The model under review builds one solid part; all positions refer to its coordinate system, in mm. Coordinates: 2 decimals unless noted, no trailing zeros. Loops run counter-clockwise (first coordinate to the right, second up) from the corner with the lowest first, then second, coordinate; pieces in that order, holes last. Notation, with made-up numbers: M -30.75,43.5 L -6.75,43.5 A21 ccw -6.75,58.5 Z; hole C 73.25,63.25 d1. An arc over 180 degrees is marked long. Use one line per item in the form item = value.
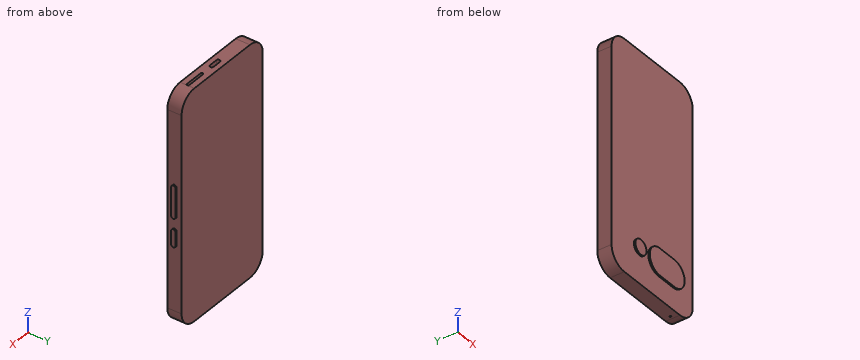
Autodesk Inventor part; units mm, degrees
ref_plane "YZ Plane" through (0, 0, 0) normal (1, 0, 0) x (0, 1, 0)
ref_plane "XZ Plane" through (0, 0, 0) normal (0, 1, 0) x (-1, 0, 0)
ref_plane "XY Plane" through (0, 0, 0) normal (0, 0, 1) x (1, 0, 0)
sketch "スケッチ1" plane through (0, 0, 0) normal (0, 1, 0) x (-1, 0, 0)
  line L0 (11.5, 0) -> (61.8, 0)
  line L1 (73.3, -11.5) -> (73.3, -143.2)
  line L2 (61.8, -154.7) -> (11.5, -154.7)
  line L3 (0, -143.2) -> (0, -11.5)
  arc A0 (73.3, -11.5) -> (61.8, 0) centre (61.8, -11.5) ccw
  arc A1 (11.5, 0) -> (0, -11.5) centre (11.5, -11.5) ccw
  arc A2 (0, -143.2) -> (11.5, -154.7) centre (11.5, -143.2) ccw
  arc A3 (61.8, -154.7) -> (73.3, -143.2) centre (61.8, -143.2) ccw
  point P0 (0, 0)
  point P1 (73.3, -154.7)
  point P2 (73.3, 0)
  point P3 (0, -154.7)
  dimension "d0" = 73.3
  dimension "d1" = 154.7
  dimension "d2" = 171.187
  dimension "d3" = 11.5
extrude "押し出し1" add sketch "スケッチ1" along normal blind 9.6
sketch "スケッチ2" plane through (-61.8, 0, 0) normal (0, 0, 1) x (1, 0, 0)
  line L0 (28.075, 6.05) -> (22.225, 6.05)
  line L1 (20.975, 4.8) -> (20.975, 4.8)
  line L2 (22.225, 3.55) -> (28.075, 3.55)
  line L3 (29.325, 4.8) -> (29.325, 4.8)
  line L4 (0, 9.6) -> (50.3, 9.6)
  line L5 (50.3, 0) -> (50.3, 9.6)
  arc A0 (22.225, 6.05) -> (20.975, 4.8) centre (22.225, 4.8) ccw
  arc A1 (20.975, 4.8) -> (22.225, 3.55) centre (22.225, 4.8) ccw
  arc A2 (28.075, 3.55) -> (29.325, 4.8) centre (28.075, 4.8) ccw
  arc A3 (29.325, 4.8) -> (28.075, 6.05) centre (28.075, 4.8) ccw
  line L6 (37.15, 5.625) -> (49.4, 5.625)
  line L7 (50.225, 4.8) -> (50.225, 4.8)
  line L8 (49.4, 3.975) -> (37.15, 3.975)
  line L9 (36.325, 4.8) -> (36.325, 4.8)
  arc A4 (50.225, 4.8) -> (49.4, 5.625) centre (49.4, 4.8) ccw
  arc A5 (49.4, 3.975) -> (50.225, 4.8) centre (49.4, 4.8) ccw
  arc A6 (37.15, 5.625) -> (36.325, 4.8) centre (37.15, 4.8) ccw
  arc A7 (36.325, 4.8) -> (37.15, 3.975) centre (37.15, 4.8) ccw
  point P0 (61.8, 0)
  point P1 (29.325, 6.05)
  point P2 (20.975, 3.55)
  point P3 (29.325, 3.55)
  point P4 (25.15, 6.05)
  point P5 (25.15, 9.6)
  point P6 (50.3, 4.8)
  point P7 (50.3, 4.8)
  point P8 (20.975, 4.8)
  point P9 (29.325, 4.8)
  point P10 (50.225, 3.975)
  point P11 (50.225, 5.625)
  point P12 (36.325, 3.975)
  point P13 (50.3, 4.8)
  point P14 (36.325, 4.8)
  point P15 (50.225, 4.8)
  dimension "d6" = 8.35
  dimension "d7" = 2.5
  dimension "d8" = 1.25
  dimension "d16" = 13.9
  dimension "d17" = 1.65
  dimension "d18" = 0.825
  dimension "d19" = 7
extrude "押し出し2" cut sketch "スケッチ2" against normal blind 5
sketch "スケッチ4" plane through (0, 0, -11.5) normal (1, 0, 0) x (0, 0, -1)
  line L0 (78.5, 6.3) -> (87.5, 6.3)
  line L1 (89, 4.8) -> (89, 4.8)
  line L2 (87.5, 3.3) -> (78.5, 3.3)
  line L3 (77, 4.8) -> (77, 4.8)
  line L4 (131.7, 0) -> (131.7, 9.6)
  arc A0 (78.5, 6.3) -> (77, 4.8) centre (78.5, 4.8) ccw
  arc A1 (77, 4.8) -> (78.5, 3.3) centre (78.5, 4.8) ccw
  arc A2 (87.5, 3.3) -> (89, 4.8) centre (87.5, 4.8) ccw
  arc A3 (89, 4.8) -> (87.5, 6.3) centre (87.5, 4.8) ccw
  line L5 (49.5, 6.3) -> (68.5, 6.3)
  line L6 (70, 4.8) -> (70, 4.8)
  line L7 (68.5, 3.3) -> (49.5, 3.3)
  line L8 (48, 4.8) -> (48, 4.8)
  arc A4 (49.5, 6.3) -> (48, 4.8) centre (49.5, 4.8) ccw
  arc A5 (48, 4.8) -> (49.5, 3.3) centre (49.5, 4.8) ccw
  arc A6 (70, 4.8) -> (68.5, 6.3) centre (68.5, 4.8) ccw
  arc A7 (68.5, 3.3) -> (70, 4.8) centre (68.5, 4.8) ccw
  point P0 (-11.5, 0)
  point P1 (89, 3.3)
  point P2 (89, 6.3)
  point P3 (77, 3.3)
  point P4 (89, 4.8)
  point P5 (131.7, 4.8)
  point P6 (70, 3.3)
  point P7 (70, 6.3)
  point P8 (48, 3.3)
  point P9 (48, 4.8)
  point P10 (70, 4.8)
  point P11 (77, 4.8)
  dimension "d20" = 12
  dimension "d21" = 3
  dimension "d22" = 42.7
  dimension "d23" = 1.5
  dimension "d24" = 22
  dimension "d25" = 7
  dimension "d26" = 3
  dimension "d27" = 1.5
extrude "押し出し3" add sketch "スケッチ4" along normal blind 1
sketch "スケッチ5" plane through (-11.5, 0, -154.7) normal (0, 0, -1) x (-1, 0, 0)
  circle A0 centre (2.15, 4.8) radius 0.5
  line L0 (0, 0) -> (0, 9.6)
  line L1 (0, 9.6) -> (50.3, 9.6)
  point P0 (-11.5, 0)
  point P1 (0, 4.8)
  point P2 (25.15, 9.6)
  dimension "d30" = 1
  dimension "d31" = 23
extrude "押し出し4" cut sketch "スケッチ5" against normal blind 5
sketch "スケッチ6" plane through (0, 0, 0) normal (0, -1, 0) x (1, 0, 0)
  line L0 (-17.6, -139.95) -> (-31.1, -139.95)
  line L1 (-40.1, -130.95) -> (-40.1, -130.95)
  line L2 (-31.1, -121.95) -> (-17.6, -121.95)
  line L3 (-8.6, -130.95) -> (-8.6, -130.95)
  line L4 (-11.5, -154.7) -> (-61.8, -154.7)
  line L5 (0, -11.5) -> (0, -143.2)
  arc A0 (-17.6, -139.95) -> (-8.6, -130.95) centre (-17.6, -130.95) ccw
  arc A1 (-8.6, -130.95) -> (-17.6, -121.95) centre (-17.6, -130.95) ccw
  arc A2 (-31.1, -121.95) -> (-40.1, -130.95) centre (-31.1, -130.95) ccw
  arc A3 (-40.1, -130.95) -> (-31.1, -139.95) centre (-31.1, -130.95) ccw
  circle A4 centre (-48.1, -130.95) radius 5
  point P0 (0, 0)
  point P1 (-40.1, -121.95)
  point P2 (-40.1, -139.95)
  point P3 (-8.6, -121.95)
  dimension "d34" = 31.5
  dimension "d35" = 18
  dimension "d36" = 14.75
  dimension "d37" = 8.6
  dimension "d38" = 9
  dimension "d41" = 10
  dimension "d43" = 8
extrude "押し出し5" add sketch "スケッチ6" along normal blind 1
properties part number "smartphone"
1. Add section D-D (x = -5). State the section outline as (y, z) points, then the cut area to 3 significant figures.
Response values:
outline = M 0,-152.69 L 9.6,-152.69 L 9.6,-2.01 L 0,-2.01 Z
area = 1,450 mm^2
2. Add section A-A (z = -66). State the section outline as (x, y) points, then the cut area to 3 significant figures.
Response values:
outline = M -73.3,0 L 0,0 L 0,3.3 L 1,3.3 L 1,6.3 L 0,6.3 L 0,9.6 L -73.3,9.6 Z
area = 707 mm^2
3. Insertion check: P1, Ø0.5, axis at x = -27, y = -0.5, coming from the +Z side; P2, Ø1.5, axis at x = -36, z = -2.5, coming from the -Y side; P3, Ø0.5, axis at x = -21.5, y = -0.5, coming from the -Z side. Each pin has a flat end and moves straight along its axis. Give the tip position at first contact, or say it passes through.
Response values:
P1 = -121.95
P2 = 0
P3 = -139.95
4. Add section C-C (z = -130.95). State the section outline as (x, y) points, then the cut area to 3 significant figures.
Response values:
outline = M -73.3,0 L -53.1,0 L -53.1,-1 L -43.1,-1 L -43.1,0 L -40.1,0 L -40.1,-1 L -8.6,-1 L -8.6,0 L 0,0 L 0,9.6 L -73.3,9.6 Z
area = 745 mm^2
5. Wall thickness on line 1 along Y through (x, z) = (-13.65, -151.45); line 2 along Y through (x, z) = (-7, -131); line 3 along X through (y, z) = (8.25, -115.5): over which ranges is each line inside the solid? List them lowest first. Write a range as from..to.
Response values:
line_1 = 0..4.3, 5.3..9.6
line_2 = 0..9.6
line_3 = -73.3..0
6. Add section B-B (y = 8). State the section outline as (x, z) points, then the cut area to 3 significant figures.
Response values:
outline = M -73.3,-143.2 A11.5 ccw -61.8,-154.7 L -11.5,-154.7 A11.5 ccw 0,-143.2 L 0,-11.5 A11.5 ccw -11.5,0 L -61.8,0 A11.5 ccw -73.3,-11.5 Z
area = 11,200 mm^2
